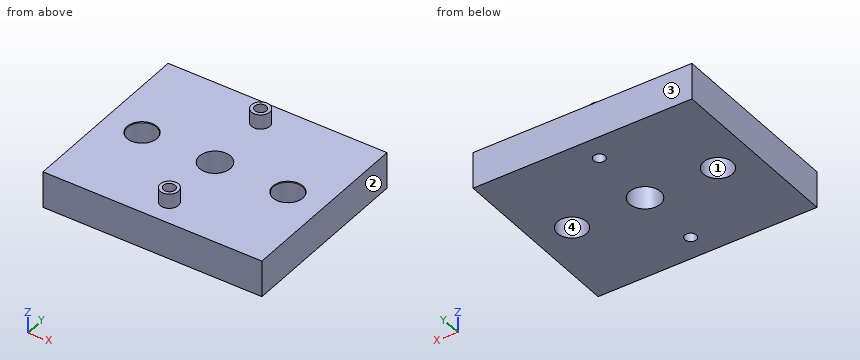
```python
from build123d import *

# Parameters (mm, degrees)
SKETCH_1_W                = 60
SKETCH_1_H                = 50
EXTRUDE_1_DEPTH           = 10
HOLE_WIZARD_1_D           = 8.5
HOLE_WIZARD_1_DEPTH       = 20
HOLE_WIZARD_2_D           = 8
HOLE_WIZARD_2_CSINK_D     = 8.2
HOLE_WIZARD_2_CSINK_ANGLE = 45
SKETCH_9_R                = 2.5
EXTRUDE_3_DEPTH           = 4
HOLE_WIZARD_3_D           = 3.2


with BuildPart() as part:
    # 草图1 → 凸台-拉伸1 (new body)
    with BuildSketch(Plane.XY):
        Rectangle(SKETCH_1_W, SKETCH_1_H)
    extrude(amount=EXTRUDE_1_DEPTH)

    # 孔1
    with Locations(Plane.XY.offset(10)):
        with Locations((0, 0)):
            Hole(HOLE_WIZARD_1_D / 2, depth=HOLE_WIZARD_1_DEPTH)

    # 孔2 (through all)
    with Locations(Plane.XY.offset(10)):
        with Locations((20, 0), (-20, 0)):
            CounterSinkHole(HOLE_WIZARD_2_D / 2, HOLE_WIZARD_2_CSINK_D / 2, counter_sink_angle=HOLE_WIZARD_2_CSINK_ANGLE)

    # 草图9 → 凸台-拉伸3 (add)
    with BuildSketch(Plane.XY.offset(10)):
        with Locations(Location((0, 18.25, 0), (0, 0, 180))):
            Circle(SKETCH_9_R)
        with Locations(Location((0, -18.25, 0), (0, 0, 180))):
            Circle(SKETCH_9_R)
    extrude(amount=EXTRUDE_3_DEPTH)

    # 孔3 (through all)
    with Locations(Plane.XY.offset(14)):
        with Locations((0, 18.25), (0, -18.25)):
            Hole(HOLE_WIZARD_3_D / 2)


solid = part.part
```
The listing builds one solid part. Answer for the finished solid, in the listing's coordinates (mm). Face numbers are marked on the shaded views. Round coordinates to 2 decimals unless told otherwise and drop trailing zeros. Write each loop counter-clockwise with the first axis right and the second up, starting at its lowest first coordinate (ties: lowest second). Pieces come first, ordered by that corner, then holes. Notation, with made-up numbers: (-19.5, 40) -> (17.5, 40) arc R33 cw to (17.5, 73) -> close; hole circle Ø8 at (68.25, 42.5). An arc over 180 degrees is marked (long way). Answer as a JSON object with one key per item and string values. Group by question number.
Q1. This flat-tipped pin is pushed along its axis until it touches: pin 1 Ø25 at (x, y) = (-14.5, -10.5) entering from +Z. Where does it stop, or does it pass through?
Q2. Section B-B (y = 0) is taken. Write down the section's boundary in (x, z), plus the area to 3 significant figures.
Q3. Section A-A (x = 0) is taken. Write down the section's boundary in (y, z).
Q4. Determine the mould class of the marked faces 1, 2, 3 and 4 for opening direction Y: pulls with the +Y half, pulls with the -Y half, needs draft (parallel to the pull), parting line crosses it, or undercut.
Q5. Straight lines are drawn through the part: line 1 along Y through (x, z) = (0, 5); line 2 along Y through (x, z) = (20, 5.5); line 3 along X through (y, z) = (-1, 7.75). For each, find the intervals that lie inside material, in ascending order.
Q6. Section D-D (x = -20) is taken. Write down the section's boundary in (y, z), plus the area to 3 significant figures.
Q7. Section C-C (z = 11.5) is taken. Write down the section's boundary in (x, y).
Check values:
{
 "1": {"pin 1": "z = 10"},
 "2": {"outline": "(-30, 0) -> (-24, 0) -> (-24, 9.76) -> (-24.1, 10) -> (-30, 10) -> close; (-16, 0) -> (-4.25, 0) -> (-4.25, 10) -> (-15.9, 10) -> (-16, 9.76) -> close; (4.25, 0) -> (16, 0) -> (16, 9.76) -> (15.9, 10) -> (4.25, 10) -> close; (24, 0) -> (30, 0) -> (30, 10) -> (24.1, 10) -> (24, 9.76) -> close", "area": "355 mm^2"},
 "3": {"outline": "(-25, 0) -> (-19.85, 0) -> (-19.85, 14) -> (-20.75, 14) -> (-20.75, 10) -> (-25, 10) -> close; (-16.65, 0) -> (-4.25, 0) -> (-4.25, 10) -> (-15.75, 10) -> (-15.75, 14) -> (-16.65, 14) -> close; (4.25, 0) -> (16.65, 0) -> (16.65, 14) -> (15.75, 14) -> (15.75, 10) -> (4.25, 10) -> close; (19.85, 0) -> (25, 0) -> (25, 10) -> (20.75, 10) -> (20.75, 14) -> (19.85, 14) -> close"},
 "4": {"face 1": "undercut", "face 2": "needs draft", "face 3": "pulls with the +Y half", "face 4": "undercut"},
 "5": {"line 1": "-25 to -19.85, -16.65 to -4.25, 4.25 to 16.65, 19.85 to 25", "line 2": "-25 to -4, 4 to 25", "line 3": "-30 to -23.87, -16.13 to -4.13, 4.13 to 16.13, 23.87 to 30"},
 "6": {"outline": "(-25, 0) -> (-4, 0) -> (-4, 9.76) -> (-4.1, 10) -> (-25, 10) -> close; (4, 0) -> (25, 0) -> (25, 10) -> (4.1, 10) -> (4, 9.76) -> close", "area": "420 mm^2"},
 "7": {"outline": "circle Ø5 at (0, -18.25); circle Ø5 at (0, 18.25); hole circle Ø3.2 at (0, -18.25); hole circle Ø3.2 at (0, 18.25)"}
}
